Autodesk Inventor part; units mm, degrees
ref_plane "YZ Plane" through (0, 0, 0) normal (1, 0, 0) x (0, 1, 0)
ref_plane "XZ Plane" through (0, 0, 0) normal (0, 1, 0) x (-1, 0, 0)
ref_plane "XY Plane" through (0, 0, 0) normal (0, 0, 1) x (1, 0, 0)
sketch "Sketch1" plane through (0, 0, 0) normal (0, 1, 0) x (-1, 0, 0)
  line L0 (20.8788, 34.798) -> (8.1788, 34.798)
  line L1 (8.1788, 34.798) -> (8.1788, 17.7292)
  line L2 (8.1788, 17.7292) -> (20.8788, 17.7292)
  line L3 (20.8788, 17.7292) -> (20.8788, 34.798)
  point P0 (0, 0)
  dimension "d0" = 17.0688
  dimension "d1" = 12.7
extrude "Extrusion1" add sketch "Sketch1" along normal blind 2.54
sketch "Sketch2" plane through (0, 2.54, 0) normal (0, 1, 0) x (1, 0, 0)
  line L0 (-8.1788, -17.7292) -> (-20.8788, -17.7292)
  line L1 (-20.8788, -34.798) -> (-8.1788, -34.798)
  line L2 (-20.8788, -17.7292) -> (-20.8788, -34.798)
  point P0 (0, 0)
  point P1 (-14.5288, -31.623)
  point P2 (-14.5288, -20.9042)
  dimension "d5" = 3.175
  dimension "d6" = 3.175
  dimension "d14" = 6.35
  dimension "d15" = 6.35
hole "Hole1" at (-14.5288, 2.54, 31.623) at (-14.5288, 2.54, 20.9042) direction (0, -1, 0) diameter 2.2098 end through all
sketch "Sketch4" plane through (0, 2.54, 0) normal (0, 1, 0) x (1, 0, 0)
  line L0 (-8.1788, -34.798) -> (-8.1788, -17.7292)
  line L1 (-20.8788, -34.798) -> (-8.1788, -34.798)
  line L2 (-8.1788, -17.7292) -> (-11.9888, -17.7292)
  line L3 (-11.9888, -17.7292) -> (-11.9888, -34.798)
  line L4 (-11.9888, -34.798) -> (-8.1788, -34.798)
  line L5 (-8.1788, -34.798) -> (-8.1788, -17.7292)
  point P0 (0, 0)
  dimension "d16" = 3.81
extrude "Extrusion2" add sketch "Sketch4" along normal blind 22.098
sketch "Sketch5" plane through (-8.1788, 0, 34.798) normal (1, 0, 0) x (0, 0, -1)
  line L0 (0, 24.638) -> (17.0688, 24.638)
  line L1 (0, 0) -> (0, 24.638)
  line L2 (17.0688, 0) -> (17.0688, 24.638)
  point P0 (34.798, 0)
  point P1 (1.5748, 5.08)
  point P2 (14.5288, 22.098)
  dimension "d26" = 2.54
  dimension "d27" = 2.54
  dimension "d29" = 17.018
  dimension "d31" = 15.494
hole "Hole2" at (-8.1788, 5.08, 33.2232) at (-8.1788, 22.098, 20.2692) direction (-1, 0, 0) diameter 3.048 end through all
sketch "Sketch6" plane through (-8.1788, 0, 34.798) normal (1, 0, 0) x (0, 0, -1)
  circle A0 centre (1.5748, 5.08) radius 2.54
  circle A1 centre (1.5748, 5.08) radius 1.524
  point P0 (34.798, 0)
  dimension "d51" = 5.08
extrude "Extrusion3" add sketch "Sketch6" against normal up to surface (3.81 mm away)
sketch "Sketch7" plane through (-8.1788, 0, 34.798) normal (1, 0, 0) x (0, 0, -1)
  line L0 (0, 24.638) -> (17.0688, 24.638)
  line L1 (0, 24.638) -> (8.1534, 24.638)
  line L2 (8.1534, 24.638) -> (8.1534, 15.0368)
  line L3 (8.1534, 15.0368) -> (0, 15.0368)
  line L4 (0, 15.0368) -> (0, 24.638)
  line L5 (17.0688, 0) -> (17.0688, 24.638)
  line L6 (0, 7.0729) -> (0, 24.638)
  dimension "d44" = 9.6012
  dimension "d46" = 8.9154
extrude "Extrusion4" cut sketch "Sketch7" against normal blind 22.098
properties part number "Ultrasonic MoUnt"
Verification items for the finished model (mm, model axes). A direction names the side the tool comes from. Round coordinates to 2 decimals unless told otherwise and drop trailing zeros. Write each loop counter-clockwise with the first axis right and the second up, starting at its lowest first coordinate (ties: lowest second). Pieces come first, ordered by that corner, then holes. Notation, with made-up numbers: (18.25, 82.5) -> (60.25, 82.5) arc R12 cw to (60.25, 105.5) -> close; hole circle Ø9 at (41, -36.5). An arc over 180 degrees is marked (long way). Write each question's results on one line, items separated by ' | '. Start each with the question number.
1. Set-up check for faces 1 (the flat face through (-15, 1, 34.798)), 2 (the flat face through (-8.179, 9, 25)), 3 (the flat face through (-11.989, 11, 25)), 4 (the flat face through (-10, 15.037, 31)), 5 (the flat face through (-11.6, 9.4, 17.729)): record each of +Z, -Z, +X, -X, +Y, -Y from which the full face is reachable in a straight line by a thin tool's end or side.
2. Cross-section at B-B (x = -15). Enter the section's corners in (y, z), then the cut area to 3 significant figures.
3. Cross-section at A-A (y = 5.08). Enter the section's corners in (x, z), then the cut area to 3 significant figures.
4. Depth check by flat-ended pin: P1, Ø2, axis at x = -14.5, z = 24, coming from the -Y side; P2, Ø4.5, axis at x = -17, z = 27, coming from the +Y side; P3, Ø10, axis at y = 10.5, z = 21.5, coming from the -X side; P4, Ø3, axis at x = -9.5, y = 9.5, coming from the +Z side. Enter the tip coordinate at first touch or a pass-through.
5. Cross-section at D-D (x = -11.5). Enter the section's corners in (y, z).
6. Draft check along Y on faces 6 (the cylindrical face through (-10.11, 4.62, 31.77)), 7 (the flat face through (-14, 0, 26)), 8 (the cylindrical face through (-10.11, 23.45, 19.57)), 9 (the cylindrical face through (-15.276, 1.252, 30.809)). Enter one of: +Y half, -Y half, draft (parallel to the pull), parting line (faces both ways), or undercut.
7. Material ranges on probe 1 along Y at (x, z) = (-14.25, 27.5); probe 2 along X at (y, z) = (12, 31); probe 3 along Z at (x, y) = (-10.85, 5.08), recorded low to high. Write a range as from..to.
8. Cross-section at C-C (z = 33.5). Enter the section's corners in (x, y).
Solutions:
1) face 1: +Z, +X, -X, -Y | face 2: +Z, -Z, +X, +Y, -Y | face 3: +Z, -Z, -X, +Y | face 4: +Z, +X, -X, +Y | face 5: -Z, +X, -X, +Y, -Y
2) outline: (0, 17.73) -> (2.54, 17.73) -> (2.54, 19.9) -> (0, 19.9) -> close; (0, 21.9) -> (2.54, 21.9) -> (2.54, 30.62) -> (0, 30.62) -> close; (0, 32.62) -> (2.54, 32.62) -> (2.54, 34.8) -> (0, 34.8) -> close | area: 33.2 mm2
3) outline: (-11.99, 17.73) -> (-8.18, 17.73) -> (-8.18, 31.7) -> (-11.99, 31.7) -> close; (-11.99, 34.75) -> (-8.18, 34.75) -> (-8.18, 35.76) -> (-11.99, 35.76) -> close | area: 57.1 mm2
4) P1: stops at y = 0 | P2: stops at y = 2.54 | P3: stops at x = -11.99 | P4: stops at z = 34.8
5) outline: (0, 17.73) -> (24.64, 17.73) -> (24.64, 26.64) -> (15.04, 26.64) -> (15.04, 34.8) -> (7.07, 34.8) arc R2.54 ccw to (3.09, 34.8) -> (0, 34.8) -> close; hole circle Ø3.05 at (5.08, 33.22); hole circle Ø3.05 at (22.1, 20.27)
6) face 6: undercut | face 7: -Y half | face 8: undercut | face 9: draft
7) probe 1: y = 0..2.54 | probe 2: x = -11.99..-8.18 | probe 3: z = 17.73..31.7, 34.75..35.76
8) outline: (-20.88, 0) -> (-8.18, 0) -> (-8.18, 3.58) -> (-11.99, 3.58) -> (-11.99, 2.54) -> (-20.88, 2.54) -> close; (-11.99, 6.58) -> (-8.18, 6.58) -> (-8.18, 15.04) -> (-11.99, 15.04) -> close
